The model under review builds one solid part; all positions refer to its coordinate system, in mm. A direction names the side the tool comes from. Coordinates: 2 decimals unless noted, no trailing zeros. Write each loop counter-clockwise with the first axis right and the second up, starting at its lowest first coordinate (ties: lowest second). Pieces come first, ordered by that corner, then holes.
```python
from build123d import *

# Parameters (mm, degrees)
SKICA1_R                 = 5
P_IDAT_VYSUNUT_M1_DEPTH  = 23.6
SKICA2_OUTSIDE_W         = 17.502
SKICA2_OUTSIDE_H         = 17.502
SKICA2_OUTSIDE_W_2       = 8.2
SKICA2_OUTSIDE_H_2       = 8.2
ODEBRAT_VYSUNUT_M1_DEPTH = 8
SKICA3_R                 = 2.5
P_IDAT_VYSUNUT_M2_DEPTH  = 2
SKICA4_R                 = 1.15
ODEBRAT_VYSUNUT_M2_DEPTH = 11
ZAOBLIT1_R               = 1


with BuildPart() as part:
    # Skica1 → Přidat vysunutím1 (new body)
    with BuildSketch(Plane.XY):
        Circle(SKICA1_R)
    extrude(amount=P_IDAT_VYSUNUT_M1_DEPTH)

    # Skica2 outside → Odebrat vysunutím1 (cut)
    with BuildSketch(Plane(origin=(0, 0, 23.6), x_dir=(-1, 0, 0), z_dir=(0, 0, -1))):
        Rectangle(SKICA2_OUTSIDE_W, SKICA2_OUTSIDE_H)
        Rectangle(SKICA2_OUTSIDE_W_2, SKICA2_OUTSIDE_H_2, mode=Mode.SUBTRACT)
    extrude(amount=ODEBRAT_VYSUNUT_M1_DEPTH, mode=Mode.SUBTRACT)

    # Skica3 → Přidat vysunutím2 (add)
    with BuildSketch(Plane.XY.offset(23.6)):
        Circle(SKICA3_R)
    extrude(amount=P_IDAT_VYSUNUT_M2_DEPTH)

    # Skica4 → Odebrat vysunutím2 (cut)
    with BuildSketch(Plane.XY.offset(25.6)):
        Circle(SKICA4_R)
    extrude(amount=-ODEBRAT_VYSUNUT_M2_DEPTH, mode=Mode.SUBTRACT)

    # Zaoblit1
    # the kernel refuses this fillet: 1 mm, written as the material it adds along each edge
    with BuildSketch(Plane(origin=(0, 0, 14.6), x_dir=(1, 0, 0), z_dir=(0, -1, 0))) as zaoblit1_piece_1:
        with BuildLine():
            CenterArc((1.15 - ZAOBLIT1_R, ZAOBLIT1_R), ZAOBLIT1_R, 270, 90)
            Line((1.15 - ZAOBLIT1_R, 0), (1.15, 0))
            Line((1.15, 0), (1.15, ZAOBLIT1_R))
        make_face()
    revolve(axis=Axis((0, 0, 14.6), (0, 0, 1)))
    # the kernel refuses this fillet: 1 mm, written as the material it takes off along each edge
    with BuildSketch(Plane(origin=(0, 0, 0), x_dir=(1, 0, 0), z_dir=(0, -1, 0))) as zaoblit1_2_piece_1:
        with BuildLine():
            CenterArc((5 - ZAOBLIT1_R, ZAOBLIT1_R), ZAOBLIT1_R, 270, 90)
            Line((5 - ZAOBLIT1_R, 0), (5, 0))
            Line((5, 0), (5, ZAOBLIT1_R))
        make_face()
    revolve(axis=Axis((0, 0, 0), (0, 0, 1)), mode=Mode.SUBTRACT)
    with BuildSketch(Plane(origin=(0, 0, 23.6), x_dir=(0.9940244909072117, 0.109157278624279, 0), z_dir=(0.109157278624279, -0.9940244909072117, 0))) as zaoblit1_2_piece_2:
        with BuildLine():
            CenterArc((5 - ZAOBLIT1_R, -ZAOBLIT1_R), ZAOBLIT1_R, 0, 90)
            Line((5 - ZAOBLIT1_R, 0), (5, 0))
            Line((5, 0), (5, -ZAOBLIT1_R))
        make_face()
    revolve(axis=Axis((0, 0, 23.6), (0, 0, 1)), revolution_arc=77.466522668, mode=Mode.SUBTRACT)
    with BuildSketch(Plane(origin=(0, 0, 23.6), x_dir=(-0.10915727862431812, 0.9940244909072075, 0), z_dir=(0.9940244909072075, 0.10915727862431812, 0))) as zaoblit1_2_piece_3:
        with BuildLine():
            CenterArc((5 - ZAOBLIT1_R, -ZAOBLIT1_R), ZAOBLIT1_R, 0, 90)
            Line((5 - ZAOBLIT1_R, 0), (5, 0))
            Line((5, 0), (5, -ZAOBLIT1_R))
        make_face()
    revolve(axis=Axis((0, 0, 23.6), (0, 0, 1)), revolution_arc=77.466522668, mode=Mode.SUBTRACT)
    with BuildSketch(Plane(origin=(0, 0, 23.6), x_dir=(-0.9940244909072075, -0.1091572786243185, 0), z_dir=(-0.1091572786243185, 0.9940244909072075, 0))) as zaoblit1_2_piece_4:
        with BuildLine():
            CenterArc((5 - ZAOBLIT1_R, -ZAOBLIT1_R), ZAOBLIT1_R, 0, 90)
            Line((5 - ZAOBLIT1_R, 0), (5, 0))
            Line((5, 0), (5, -ZAOBLIT1_R))
        make_face()
    revolve(axis=Axis((0, 0, 23.6), (0, 0, 1)), revolution_arc=77.466522668, mode=Mode.SUBTRACT)
    with BuildSketch(Plane(origin=(0, 0, 23.6), x_dir=(0.10915727862436878, -0.9940244909072019, 0), z_dir=(-0.9940244909072019, -0.10915727862436878, 0))) as zaoblit1_2_piece_5:
        with BuildLine():
            CenterArc((5 - ZAOBLIT1_R, -ZAOBLIT1_R), ZAOBLIT1_R, 0, 90)
            Line((5 - ZAOBLIT1_R, 0), (5, 0))
            Line((5, 0), (5, -ZAOBLIT1_R))
        make_face()
    revolve(axis=Axis((0, 0, 23.6), (0, 0, 1)), revolution_arc=77.466522668, mode=Mode.SUBTRACT)
    with BuildSketch(Plane(origin=(5.361817604, -4.1, 23.6), x_dir=(0, 1, 0), z_dir=(-1, 0, 0)), Plane(origin=(-5.361817604, 4.1, 23.6), x_dir=(0, -1, 0), z_dir=(1, 0, 0)), Plane(origin=(-4.1, -5.361817604, 23.6), x_dir=(1, 0, 0), z_dir=(0, 1, 0))) as zaoblit1_2_piece_6:
        with BuildLine():
            CenterArc((ZAOBLIT1_R, ZAOBLIT1_R), ZAOBLIT1_R, 180, 90)
            Line((0, ZAOBLIT1_R), (0, 0))
            Line((0, 0), (ZAOBLIT1_R, 0))
        make_face()
    extrude(amount=10.723635209, mode=Mode.SUBTRACT)
    with BuildSketch(Plane(origin=(4.1, 5.361817604, 23.6), x_dir=(0, 0, -1), z_dir=(0, -1, 0))) as zaoblit1_2_piece_7:
        with BuildLine():
            CenterArc((ZAOBLIT1_R, -ZAOBLIT1_R), ZAOBLIT1_R, 90, 90)
            Line((0, -ZAOBLIT1_R), (0, 0))
            Line((0, 0), (ZAOBLIT1_R, 0))
        make_face()
    extrude(amount=10.723635209, mode=Mode.SUBTRACT)


solid = part.part
```
Item 1: Take a section at A-A, the plane z = 22. Write out the cut boundary in (x, y).
Solved:
outline: (-4.1, -2.86) arc R5 ccw to (-2.86, -4.1) - (2.86, -4.1) arc R5 ccw to (4.1, -2.86) - (4.1, 2.86) arc R5 ccw to (2.86, 4.1) - (-2.86, 4.1) arc R5 ccw to (-4.1, 2.86) - close; hole circle Ø2.3 at (0, 0)
Item 2: For pin 1 (4 mm diameter, centred on x = -3, z = 15, fed in from -Y); pin 2 (3 mm diameter, centred on x = -0.5, z = 18.5, fed in from -Y); pin 3 (0.5 mm diameter, centred on x = 1.5, y = 4.5, fed in from +Z), all flat-tipped, find the tip position at first contact; note any pin that passes through.
Solved:
pin 1: stops at y = -4.9
pin 2: stops at y = -4.1
pin 3: stops at z = 15.6
Item 3: To check wall thickness, follow line 1 along Y through (x, z) = (0, 20.75); line 2 along Z through (x, y) = (2.5, 2.5); line 3 along Y through (x, z) = (-0.5, 18.75). State the ranges of each line that lie inside material, in increasing order.
Solved:
line 1: y = -4.1 to -1.15, 1.15 to 4.1
line 2: z = 0 to 23.6
line 3: y = -4.1 to -1.04, 1.04 to 4.1
Item 4: Machinability: for faces 1 (the face through (4.1, 0, 19)), 2 (the face through (0, 4.1, 19)), 3 (the face through (-4.1, 0, 19)), which of the approach directions +Z, -Z, +X, -X, +Y, -Y give a long, thin tool a straight path to every point of the face, cutting with its end or side? Answer none if there is none.
Solved:
face 1: +Z, +X, +Y, -Y
face 2: +Z, +X, -X, +Y
face 3: +Z, -X, +Y, -Y
Item 5: Mouldability with a two-part tool opening along Y and no side actions: class faces 4 (the face through (-0.91, -0.7, 20.67)), 5 (the face through (-0.54, -2.44, 24.59)), 6 (the face through (0, -4.1, 19)), 7 (the face through (1, -1, 25.6)) as pulls with the +Y half, pulls with the -Y half, needs draft (parallel to the pull), parting line crosses it, or undercut.
Solved:
face 4: undercut
face 5: parting line crosses it
face 6: pulls with the -Y half
face 7: needs draft
